Here's how the part is built. I have some questions about the finished solid (model axes, mm). Face numbers are marked on the shaded views. A direction names the side the tool comes from. Coordinates: 2 decimals unless noted, no trailing zeros. Write each loop counter-clockwise with the first axis right and the second up, starting at its lowest first coordinate (ties: lowest second). Pieces come first, ordered by that corner, then holes. Notation, with made-up numbers: (-33.5, 57) -> (-7.5, 57) arc R9 cw to (-7.5, 62) -> close; hole circle Ø6 at (55, 7). An arc over 180 degrees is marked (long way). Use a Markdown table: item, result. Add a question column.
Item 1: If I drill on line 1 along X through (y, z) = (1, 14); line 2 along Z through (x, y) = (-16.5, 2.25); line 3 along Y through (x, z) = (-39, 10.25), over which ranges is the centre line in solid material (lowest first)? Write a range as from..to.
Item 2: Imagine slicing it at D-D, the plane x = -29. Write out the boundary of the cut face in (y, z), and give its area (3 significant figures).
Item 3: On a 3-axis mill with a long thin cutter (end or side, diameter ignored), from which of +Z, -Z, +X, -X, +Y, -Y can I reach the whole of each face in a straight line? I mean the marked faces 1, 2, 3 and 4. Say none if no direction works.
Item 4: Imagine slicing it at A-A, the plane x = 15.5. Write out the boundary of the cut face in (y, z), and give its area (3 significant figures).
Item 5: Imagine slicing it at C-C, the plane z = 9.5. Write out the boundary of the cut face in (x, y).
Item 6: Imagine slicing it at B-B, the plane y = -1.5. Write out the boundary of the cut face in (x, z).
Item 7: Will these pins go through, and if not, where does the flat tip stop? pin 1 Ø5 at (x, z) = (-22, 9) entering from -Y; pin 2 Ø4 at (x, y) = (-26.5, -1) entering from +Z; pin 3 Ø6 at (x, z) = (-7, 13) entering from +Y.
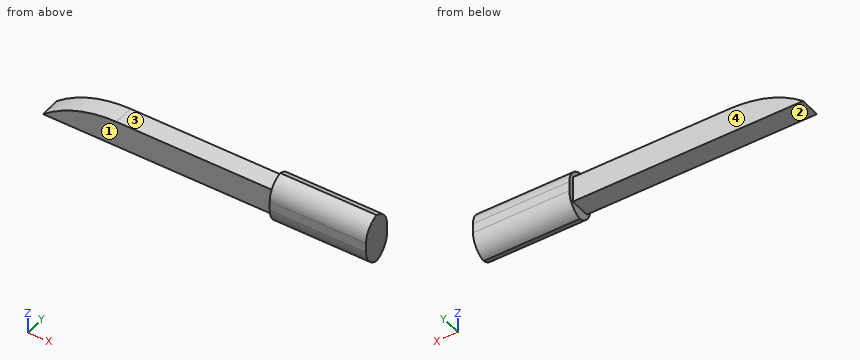
```python
from build123d import *

# Parameters (mm, degrees)
F1_DEPTH    = 2.54
F2_DEPTH    = 3.81
F3_T1_DEPTH = 49.3776003865


# Not quite as in the source:
# - a fillet or chamfer that OpenCascade refuses, or shapes differently, is made with other operations: its cross-section is extruded or revolved along the edge and cut away or added


with BuildPart() as f1:
    # F0 (on Front) → F1 (new body, symmetric)
    with BuildSketch(Plane.XZ):
        with BuildLine():
            ThreePointArc((-36.8458546815, 12.765225481), (-46.5506501675, 11.0912601627), (-55.133856614, 6.2628253844))
            Line((-55.133856614, 6.2628253844), (2.168544932, 6.2628253844))
            Line((2.168544932, 6.2628253844), (2.168544932, 9.5140254327))
            Line((2.168544932, 9.5140254327), (2.168544932, 12.765225481))
            Line((2.168544932, 12.765225481), (-36.8458546815, 12.765225481))
        make_face()
    extrude(amount=F1_DEPTH, both=True)

    # F0 (on Front) → F2 (join, symmetric)
    with BuildSketch(Plane.XZ):
        Polygon((2.168544932, 9.5140254327), (2.168544932, 6.2628253844), (2.168544932, 3.2148253844), (26.1461453185, 3.2148253844), (26.1461453185, 9.5140254327), align=None)
        Polygon((2.168544932, 12.765225481), (2.168544932, 9.5140254327), (26.1461453185, 9.5140254327), (26.1461453185, 15.813225481), (2.168544932, 15.813225481), align=None)
    extrude(amount=F2_DEPTH, both=True)

    # F3: fillet of radius 5.08 on 4 edges, made by hand

    # F3_s2 → F3_t1 (cut)
    with BuildSketch(Plane.YZ.offset(-10.531455068)):
        with BuildLine():
            ThreePointArc((-3.81, 10.733225481), (-2.3221024484, 14.3253279294), (1.27, 15.813225481))
            Line((1.27, 15.813225481), (-3.81, 15.813225481))
            Line((-3.81, 15.813225481), (-3.81, 10.733225481))
        make_face()
        with BuildLine():
            ThreePointArc((1.27, 3.2148253844), (-2.3221024484, 4.7027229359), (-3.81, 8.2948253844))
            Line((-3.81, 8.2948253844), (-3.81, 3.2148253844))
            Line((-3.81, 3.2148253844), (1.27, 3.2148253844))
        make_face()
        with BuildLine():
            ThreePointArc((3.81, 10.733225481), (2.3221024484, 14.3253279294), (-1.27, 15.813225481))
            Line((-1.27, 15.813225481), (3.81, 15.813225481))
            Line((3.81, 15.813225481), (3.81, 10.733225481))
        make_face()
        with BuildLine():
            ThreePointArc((-1.27, 3.2148253844), (2.3221024484, 4.7027229359), (3.81, 8.2948253844))
            Line((3.81, 8.2948253844), (3.81, 3.2148253844))
            Line((3.81, 3.2148253844), (-1.27, 3.2148253844))
        make_face()
    extrude(amount=F3_T1_DEPTH, mode=Mode.SUBTRACT)


solid = f1.part
```
Ans:
| question | item | result |
|---|---|---|
| 1 | line 1 | x = 2.17..26.15 |
| 1 | line 2 | z = 6.26..12.77 |
| 1 | line 3 | y = -2.54..2.54 |
| 2 | outline | (-2.54, 6.26) -> (2.54, 6.26) -> (2.54, 12.77) -> (-2.54, 12.77) -> close |
| 2 | area | 33.0 mm^2 |
| 3 | face 1 | +Z, -Z, -X, -Y |
| 3 | face 2 | -Z, -X, +Y, -Y |
| 3 | face 3 | +Z, -X, +Y, -Y |
| 3 | face 4 | +Z, -Z, -X, +Y |
| 4 | outline | (-3.81, 8.29) arc R5.08 ccw to (0, 3.38) arc R5.08 ccw to (3.81, 8.29) -> (3.81, 10.73) arc R5.08 ccw to (0, 15.65) arc R5.08 ccw to (-3.81, 10.73) -> close |
| 4 | area | 74.1 mm^2 |
| 5 | outline | (-50.21, -2.54) -> (2.17, -2.54) -> (2.17, -3.81) -> (26.15, -3.81) -> (26.15, 3.81) -> (2.17, 3.81) -> (2.17, 2.54) -> (-50.21, 2.54) -> close |
| 6 | outline | (-55.13, 6.26) -> (2.17, 6.26) -> (2.17, 4.04) -> (26.15, 4.04) -> (26.15, 14.99) -> (2.17, 14.99) -> (2.17, 12.77) -> (-36.85, 12.77) arc R28.97 ccw to start |
| 7 | pin 1 | stops at y = -2.54 |
| 7 | pin 2 | stops at z = 12.77 |
| 7 | pin 3 | stops at y = 2.54 |
